from build123d import *

# Parameters (mm, degrees)
SKETCH1_R                       = 3
BOSS_EXTRUDE1_DEPTH             = 10
FILLET1_R                       = 3
CIRPATTERN1_COUNT               = 2
CIRPATTERN1_ANGLE               = 45
CIRPATTERN2_COUNT               = 2
CIRPATTERN2_ANGLE               = 45
M3_TAPPED_HOLE4_D               = 2.5
M3_TAPPED_HOLE4_DEPTH           = 7.5
M3_TAPPED_HOLE4_TIP             = 0.751075774
M3_TAPPED_HOLE4_ON_FACE_2_D     = 2.5
M3_TAPPED_HOLE4_ON_FACE_2_DEPTH = 7.5
M3_TAPPED_HOLE4_ON_FACE_2_TIP   = 0.751075774


with BuildPart() as part:
    # Sketch1 → Boss-Extrude1 (new body)
    with BuildSketch(Plane.XY):
        with BuildLine():
            ThreePointArc((35, 0), (24.748737342, 24.748737342), (0, 35))
            ThreePointArc((0, 35), (-7.687744108, 34.145257219), (-15, 31.622776602))
            Line((-15, 31.622776602), (-15, 26))
            Line((-15, 26), (0, 26))
            ThreePointArc((0, 26), (3.168421474, 25.806222222), (6.289614512, 25.227777335))
            ThreePointArc((6.289614512, 25.227777335), (20.48816704, 16.00734242), (26, 0))
            ThreePointArc((26, 0), (20.48816704, -16.00734242), (6.289614512, -25.227777335))
            ThreePointArc((6.289614512, -25.227777335), (3.168421474, -25.806222222), (0, -26))
            Line((0, -26), (-15, -26))
            Line((-15, -26), (-15, -31.622776602))
            ThreePointArc((-15, -31.622776602), (-7.687744108, -34.145257219), (0, -35))
            ThreePointArc((0, -35), (24.748737342, -24.748737342), (35, 0))
        make_face()
        with Locations((6.289614512, -29.844442519)):
            Circle(SKETCH1_R, mode=Mode.SUBTRACT)
        with Locations((30.166206258, -4.5)):
            Circle(SKETCH1_R, mode=Mode.SUBTRACT)
        with Locations((30.166206258, 4.5)):
            Circle(SKETCH1_R, mode=Mode.SUBTRACT)
        with Locations((6.289614512, 29.844442519)):
            Circle(SKETCH1_R, mode=Mode.SUBTRACT)
        with BuildLine():
            ThreePointArc((-15, 31.622776602), (-7.687744108, 34.145257219), (0, 35))
            Line((0, 35), (-15, 35))
            Line((-15, 35), (-15, 31.622776602))
        make_face()
        with BuildLine():
            Line((-15, -35), (0, -35))
            ThreePointArc((0, -35), (-7.687744108, -34.145257219), (-15, -31.622776602))
            Line((-15, -31.622776602), (-15, -35))
        make_face()
    extrude(amount=BOSS_EXTRUDE1_DEPTH)

    # Fillet1
    fillet1_edges = [part.edges().sort_by_distance(p)[0] for p in [
        (-15, 26, 5),
        (-15, 35, 5),
        (-15, -35, 5),
        (-15, -26, 5),
    ]]
    fillet(fillet1_edges, radius=FILLET1_R)

    # Sketch14 → M3 Tapped Hole3 (revolve, cut)
    with BuildSketch(Plane(origin=(35, 0, 5), x_dir=(0, 0, -1), z_dir=(0, 1, 0))):
        Polygon((0, 0), (0, 8.251075774), (1.25, 7.5), (1.25, 0), align=None)
    m3_tapped_hole3 = revolve(axis=Axis((41.35, 0, 5), (-1, 0, 0)), mode=Mode.SUBTRACT)

    # CirPattern1: M3 Tapped Hole3 ×2 about axis
    cirpattern1_axis = Axis((0, 0, 0), (0, 0, 1))
    for i in range(1, CIRPATTERN1_COUNT):
        add(m3_tapped_hole3.rotate(cirpattern1_axis, i * CIRPATTERN1_ANGLE / (CIRPATTERN1_COUNT - 1)), mode=Mode.SUBTRACT)

    # CirPattern2: M3 Tapped Hole3 ×2 about axis
    cirpattern2_axis = Axis((0, 0, 10), (0, 0, -1))
    for i in range(1, CIRPATTERN2_COUNT):
        add(m3_tapped_hole3.rotate(cirpattern2_axis, i * CIRPATTERN2_ANGLE / (CIRPATTERN2_COUNT - 1)), mode=Mode.SUBTRACT)

    # M3 Tapped Hole4
    with Locations(Plane(origin=(-5, -35, 5), x_dir=(0, 0, -1), z_dir=(0, -1, 0))):
        with Locations((0, 0)):
            Hole(M3_TAPPED_HOLE4_D / 2, depth=M3_TAPPED_HOLE4_DEPTH)
            with Locations((0, 0, -(M3_TAPPED_HOLE4_DEPTH + M3_TAPPED_HOLE4_TIP / 2))):  # 118° drill point
                Cone(0, M3_TAPPED_HOLE4_D / 2, M3_TAPPED_HOLE4_TIP, mode=Mode.SUBTRACT)

    # M3 Tapped Hole4 on face 2
    with Locations(Plane(origin=(-5, 35, 5), x_dir=(0, 0, 1), z_dir=(0, 1, 0))):
        with Locations((0, 0)):
            Hole(M3_TAPPED_HOLE4_ON_FACE_2_D / 2, depth=M3_TAPPED_HOLE4_ON_FACE_2_DEPTH)
            with Locations((0, 0, -(M3_TAPPED_HOLE4_ON_FACE_2_DEPTH + M3_TAPPED_HOLE4_ON_FACE_2_TIP / 2))):  # 118° drill point
                Cone(0, M3_TAPPED_HOLE4_ON_FACE_2_D / 2, M3_TAPPED_HOLE4_ON_FACE_2_TIP, mode=Mode.SUBTRACT)


solid = part.part
Input: part model. Units: mm. Frame: model coordinates. A direction names the side the tool comes from. Round coordinates to 2 decimals unless told otherwise and drop trailing zeros. Write each loop counter-clockwise with the first axis right and the second up, starting at its lowest first coordinate (ties: lowest second). Pieces come first, ordered by that corner, then holes.
1) Reachability of faces 1 (the flat face through (-6, -26, 5)), 2 (the cylindrical face through (-6.22, -31.2, 4.73)), 3 (the cylindrical face through (31.3, -0.38, 3.81)) from +Z, -Z, +X, -X, +Y, -Y: full face, straight path, thin tool, end or side. Return the list, or none.
2) Cut plane C-C (z = 7). Return the cut outline in (x, y), then the cut area to 3 significant figures.
3) Cut plane D-D (y = -14). Return the cut outline in (x, z), then the cut area to 3 significant figures.
4) Contact query for flat-ended pins moving along their axis: P1, Ø1, axis at x = 16.5, z = 3.5, coming from the -Y side; P2, Ø2, axis at y = 7, z = 4, coming from the -X side; P3, Ø4, axis at x = 10, z = 1.5, coming from the -Y side. Output: stop coordinate, or through.
5) Draft query along X for faces 4 (the conical face through (26.88, -0.01, 5.22)), 5 (the conical face through (19.11, 18.903, 5.16)), 6 (the cylindrical face through (-14.14, 26.9, 5.07)). Return one class per face: pulls with the +X half, pulls with the -X half, needs draft (parallel to the pull), parting line crosses it, or undercut.
6) Cut plane B-B (y = 4.5). Return the cut outline in (x, z).
7) Ray query, L1, parallel to Y at x = -3.5, z = 7.75; L2, parallel to Z at x = 32, y = 0; L3, parallel to X at y = -28, z = 6. Return the intervals inside material, ascending.
8) Cut plane A-A (x = -9). Return the cut outline in (y, z).
Geometry says:
1. face 1: +Z, -Z, -X
1. face 2: -Y
1. face 3: +X
2. outline: (-15, -32) arc R3 ccw to (-12, -35) - (0, -35) arc R35 ccw to (0, 35) - (-12, 35) arc R3 ccw to (-15, 32) - (-15, 29) arc R3 ccw to (-12, 26) - (0, 26) arc R26 cw to (0, -26) - (-12, -26) arc R3 ccw to (-15, -29) - close; hole circle Ø6 at (6.29, -29.84); hole circle Ø6 at (6.29, 29.84); hole circle Ø6 at (30.17, -4.5); hole circle Ø6 at (30.17, 4.5)
2. area: 1,010 mm2
3. outline: (21.91, 0) - (32.08, 0) - (32.08, 10) - (21.91, 10) - close
3. area: 102 mm2
4. P1: stops at y = -31.13
4. P2: stops at x = 24.74
4. P3: stops at y = -34.07
5. face 4: pulls with the +X half
5. face 5: undercut
5. face 6: pulls with the -X half
6. outline: (25.61, 0) - (27.17, 0) - (27.17, 10) - (25.61, 10) - close; (33.17, 0) - (34.71, 0) - (34.71, 10) - (33.17, 10) - close
7. L1: y = -35 to -26, 26 to 35
7. L2: z = 0 to 3.75, 6.25 to 10
7. L3: x = -14.83 to -5.75, -4.25 to 3.92, 8.66 to 21
8. outline: (-35, 0) - (-26, 0) - (-26, 10) - (-35, 10) - close; (26, 0) - (35, 0) - (35, 10) - (26, 10) - close
